For this review, take the finished solid that the model builds, in its own axes (mm). Face numbers are marked on the shaded views. A direction names the side the tool comes from. Give positions to 0.01 mm unless a question says otherwise; leave off trailing zeros. Write each loop counter-clockwise with the first axis right and the second up, starting at its lowest first coordinate (ties: lowest second). Pieces come first, ordered by that corner, then holes. Notation, with made-up numbers: (-7, 23.25) -> (-2, 23.25) arc R10 cw to (-2, 31.25) -> close; hole circle Ø9 at (6.5, -4). An arc over 180 degrees is marked (long way). Return JSON: item names as keys, results as strings.
from build123d import *

# Parameters (mm, degrees)
SKETCH_R             = 9.375
PAD_DEPTH            = 25
SKETCH001_R          = 2
POCKET_DEPTH         = 12.5
SKETCH002_R          = 4
POCKET001_DEPTH      = 12.5
BODY_PLACEMENT_ANGLE = 180


with BuildPart() as part:
    # Sketch → Pad (new body)
    with BuildSketch(Plane.XY):
        Circle(SKETCH_R)
    extrude(amount=PAD_DEPTH)

    # Sketch001 (on Face3 of Pad) → Pocket (cut)
    with BuildSketch(Plane.XY.offset(25)):
        Circle(SKETCH001_R)
    extrude(amount=-POCKET_DEPTH, mode=Mode.SUBTRACT)

    # Sketch002 (on Face2 of Pocket) → Pocket001 (cut)
    with BuildSketch(Plane(origin=(0, 0, 0), x_dir=(1, 0, 0), z_dir=(0, 0, -1))):
        Circle(SKETCH002_R)
    extrude(amount=-POCKET001_DEPTH, mode=Mode.SUBTRACT)


with BuildPart() as part_1:
    # Body placement: moved
    add(part.part.moved(Location((0, 0, 72))).rotate(Axis((0, 0, 72), (0, 1, 0)), BODY_PLACEMENT_ANGLE))


solid = part_1.part
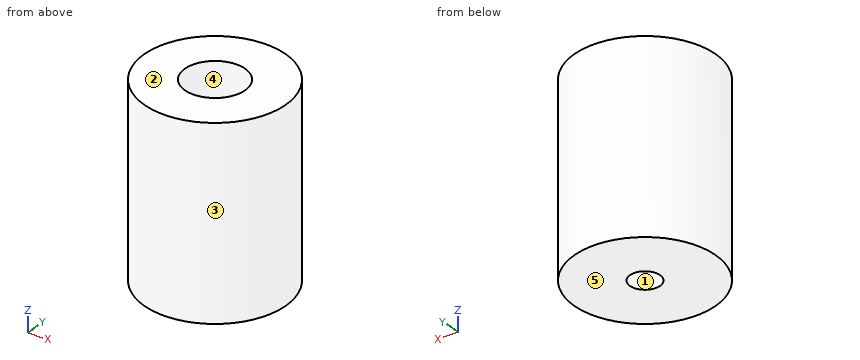
1. For the marked faces 4 and 5, list the 3-axis set-ups (+Z, -Z, +X, -X, +Y, -Y) from which the entire face can be reached by the end or side of a thin tool; tool diameter is ignored.
Results found:
{"face 4": "+Z", "face 5": "-Z, +X, -X, +Y, -Y"}
2. For pin 1 (6 mm diameter, centred on y = -4.5, z = 67, fed in from +X); pin 2 (4.5 mm diameter, centred on x = 0, y = 0, fed in from +Z); pin 3 (5 mm diameter, centred on y = -4.5, z = 64, fed in from -X), all flat-tipped, find the tip position at first contact; note any pin that passes through.
Results found:
{"pin 1": "stops at x = 9.25", "pin 2": "stops at z = 59.5", "pin 3": "stops at x = -9.16"}
3. Add section A-A, the plane x = 0. State the section outline as (y, z) points (3 decimals), plus the area to 3 significant figures.
Results found:
{"outline": "(-9.375, 47) -> (-2, 47) -> (-2, 59.5) -> (-4, 59.5) -> (-4, 72) -> (-9.375, 72) -> close; (2, 47) -> (9.375, 47) -> (9.375, 72) -> (4, 72) -> (4, 59.5) -> (2, 59.5) -> close", "area": "319 mm²"}
4. The part is to be moulded in two halves that separate along X. For the marked faces 1, 2 and 3, say which applies: +X half, -X half, draft (parallel to the pull), parting line (faces both ways), or undercut.
Results found:
{"face 1": "undercut", "face 2": "draft", "face 3": "parting line"}
5. To check wall thickness, follow probe 1 along X at (y, z) = (-0.25, 63.25); probe 2 along Y at (x, z) = (0, 51.75) (3 decimals); probe 3 along Z at (x, y) = (-2.25, -3). State the ranges of each line that lie inside material, in increasing order.
Results found:
{"probe 1": "x = -9.37 to -3.99, 3.99 to 9.37", "probe 2": "y = -9.375 to -2, 2 to 9.375", "probe 3": "z = 47 to 59.5"}
6. Add section D-D, the plane x = 8. State the section outline as (y, z) points, plus the area to 3 significant figures.
Results found:
{"outline": "(-4.89, 47) -> (4.89, 47) -> (4.89, 72) -> (-4.89, 72) -> close", "area": "244 mm²"}
7. Add section C-C, the plane z = 51.25. State the section outline as (x, y) points (3 decimals), plus the area to 3 significant figures.
Results found:
{"outline": "circle Ø18.75 at (0, 0); hole circle Ø4 at (0, 0)", "area": "264 mm²"}
